from build123d import *

# Parameters (mm, degrees)
F1_DEPTH = 60
F2_SIZE  = 10
F3_R     = 25
F4_DEPTH = 25


with BuildPart() as f1:
    # F0 (on Front) → F1 (new body)
    with BuildSketch(Plane.XZ):
        with BuildLine():
            Line((26.660392, 80.263265), (-23.339608, 80.263265))
            ThreePointArc((-23.339608, 80.263265), (-41.017278, 72.940934), (-48.339608, 55.263265))
            Line((-48.339608, 55.263265), (-48.339608, 5.263265))
            ThreePointArc((-48.339608, 5.263265), (-41.017278, -12.414405), (-23.339608, -19.736735))
            Line((-23.339608, -19.736735), (26.660392, -19.736735))
            ThreePointArc((26.660392, -19.736735), (44.338061, -12.414405), (51.660392, 5.263265))
            Line((51.660392, 5.263265), (51.660392, 55.263265))
            ThreePointArc((51.660392, 55.263265), (44.338061, 72.940934), (26.660392, 80.263265))
        make_face()
    extrude(amount=F1_DEPTH)

    # F2
    f2_edges = [f1.edges().sort_by_distance(p)[0] for p in [
        (51.660392, -60, 30.263265),
        (44.338061, -60, 72.940934),
        (1.660392, -60, 80.263265),
        (-41.017278, -60, 72.940934),
        (-48.339608, -60, 30.263265),
        (-41.017278, -60, -12.414405),
        (1.660392, -60, -19.736735),
        (44.338061, -60, -12.414405),
    ]]
    chamfer(f2_edges, length=F2_SIZE)

    # F3 (on face) → F4 (cut)
    with BuildSketch(Plane.XZ.offset(60)):
        with Locations((0, 23.312023)):
            Circle(F3_R)
    extrude(amount=-F4_DEPTH, mode=Mode.SUBTRACT)


solid = f1.part
Could you check a few things on this model? Use its own coordinates, in mm. A direction names the side the tool comes from. Give positions to 0.01 mm unless a question says otherwise; leave off trailing zeros. Order: outer loops, then holes, each group sorted by start corner. A loop starts at its lowest first (then second) coordinate and runs counter-clockwise, first axis right, second up. Notation, with made-up numbers: (80.5, 2) - (135.5, 2) arc R6 cw to (135.5, 12) - close; hole circle Ø3 at (45.5, 75). An arc over 180 degrees is marked (long way). One line per item, written item: value. Start each with the question number.
1. For faces 4 (the face through (1, 0, 31)), 5 (the face through (0, -35, 24)), which set-ups out of +Z, -Z, +X, -X, +Y, -Y let a thin tool reach every point of the face, with its end or its side?
2. Thinking about a two-plate mould opening in X: for faces 1 (the face through (46.59, -55.07, 29.91)), 2 (the face through (-40.822, -24.65, 73.134)), 3 (the face through (11.536, -47.675, 1.133)), which applies, +X half, -X half, draft (parallel to the pull), parting line (faces both ways), or undercut?
3. Imagine slicing it at B-B on x = 0. List the corners of the cut face in (y, z) for me.
4. Imagine slicing it at A-A on y = -8. List the corners of the cut face in (x, z) for me.
5. For P1, Ø10, axis at y = -18.5, z = -8, coming from the -X side; P2, Ø2, axis at x = 32.5, y = -18, coming from the +Z side, each with a flat end and sliding along its axis, tell me the tip position at first contact or that it passes through.
6. If I drill on probe 1 along Z at (x, y) = (0, -40); probe 2 along Y at (x, z) = (-8.5, 17); probe 3 along Z at (x, y) = (16, -38), over which ranges is the centre line in solid material (lowest first)?
7. Imagine slicing it at C-C on y = -47.5. List the corners of the cut face in (x, z) for me, plus the area to 3 significant figures.
8. Imagine slicing it at D-D on x = 18. List the corners of the cut face in (y, z) for me, plus the area to 3 significant figures.
Values:
1. face 4: +Z, -Z, +X, -X, +Y
1. face 5: -Y
2. face 1: +X half
2. face 2: -X half
2. face 3: undercut
3. outline: (-60, -9.74) - (-50, -19.74) - (0, -19.74) - (0, 80.26) - (-50, 80.26) - (-60, 70.26) - (-60, 48.31) - (-35, 48.31) - (-35, -1.69) - (-60, -1.69) - close
4. outline: (-48.34, 5.26) arc R25 ccw to (-23.34, -19.74) - (26.66, -19.74) arc R25 ccw to (51.66, 5.26) - (51.66, 55.26) arc R25 ccw to (26.66, 80.26) - (-23.34, 80.26) arc R25 ccw to (-48.34, 55.26) - close
5. P1: x = -46.93
5. P2: z = 79.79
6. probe 1: -19.74 to -1.69, 48.31 to 80.26
6. probe 2: -35 to 0
6. probe 3: -19.74 to 4.1, 42.52 to 80.26
7. outline: (-48.34, 5.26) arc R25 ccw to (-23.34, -19.74) - (26.66, -19.74) arc R25 ccw to (51.66, 5.26) - (51.66, 55.26) arc R25 ccw to (26.66, 80.26) - (-23.34, 80.26) arc R25 ccw to (-48.34, 55.26) - close; hole circle Ø50 at (0, 23.31)
7. area: 7,500 mm²
8. outline: (-60, -9.74) - (-50, -19.74) - (0, -19.74) - (0, 80.26) - (-50, 80.26) - (-60, 70.26) - (-60, 40.66) - (-35, 40.66) - (-35, 5.96) - (-60, 5.96) - close
8. area: 5,030 mm²
